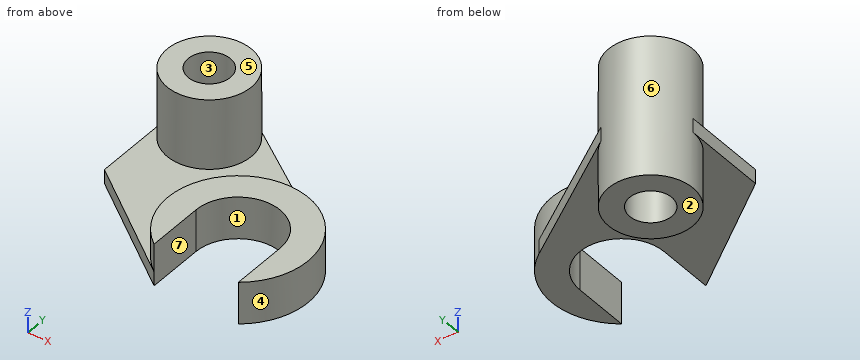
from build123d import *

# Parameters (mm, degrees)
SKETCH1_R                = 30
SKETCH1_R_2              = 15
BOSS_EXTRUDE1_DEPTH      = 50
BOSS_EXTRUDE1_DEPTH_BACK = 50
BOSS_EXTRUDE2_DEPTH      = 20
BOSS_EXTRUDE2_DEPTH_BACK = 10
BOSS_EXTRUDE3_DEPTH      = 10
SKETCH9_R                = 15
CUT_EXTRUDE1_DEPTH       = 51
CUT_EXTRUDE1_DEPTH_BACK  = 51


with BuildPart() as part:
    # Sketch1 → Boss-Extrude1 (new body, two sides)
    with BuildSketch(Plane.XY) as boss_extrude1_sk:
        Circle(SKETCH1_R)
        Circle(SKETCH1_R_2, mode=Mode.SUBTRACT)
    extrude(amount=BOSS_EXTRUDE1_DEPTH)
    extrude(boss_extrude1_sk.sketch, amount=-BOSS_EXTRUDE1_DEPTH_BACK)



with BuildPart() as body_2:
    # Sketch2 → Boss-Extrude2 (new body, two sides)
    with BuildSketch(Plane.XY) as boss_extrude2_sk:
        with BuildLine():
            Line((110, -80), (110, -120))
            ThreePointArc((110, -120), (80, -30), (50, -120))
            Line((50, -120), (50, -80))
            ThreePointArc((50, -80), (80, -50), (110, -80))
        make_face()
    extrude(amount=BOSS_EXTRUDE2_DEPTH)
    extrude(boss_extrude2_sk.sketch, amount=-BOSS_EXTRUDE2_DEPTH_BACK)


with BuildPart() as part_1:
    add(part.part)

    add(body_2.part)  # Boss-Extrude3 merges body 2
    # Sketch3 → Boss-Extrude3 (add)
    with BuildSketch(Plane.XY):
        Polygon((17.129116361, 24.629116361), (108.548527268, -38.951472732), (50, -120), (-30, -60), (-30, 0), align=None)
    extrude(amount=-BOSS_EXTRUDE3_DEPTH)

    # Sketch9 → Cut-Extrude1 (cut, two sides)
    with BuildSketch(Plane.XY) as cut_extrude1_sk:
        Circle(SKETCH9_R)
        with BuildLine():
            Line((50, -80), (50, -120))
            Line((50, -120), (110, -120))
            Line((110, -120), (110, -80))
            ThreePointArc((110, -80), (80, -50), (50, -80))
        make_face()
    extrude(amount=CUT_EXTRUDE1_DEPTH, mode=Mode.SUBTRACT)
    extrude(cut_extrude1_sk.sketch, amount=-CUT_EXTRUDE1_DEPTH_BACK, mode=Mode.SUBTRACT)


solid = part_1.part
Work out the finished part from the listing and answer in its coordinate system (mm). Face numbers are marked on the shaded views. A direction names the side the tool comes from. Give positions to 0.01 mm unless a question says otherwise; leave off trailing zeros. Order: outer loops, then holes, each group sorted by start corner. A loop starts at its lowest first (then second) coordinate and runs counter-clockwise, first axis right, second up. Notation, with made-up numbers: (39.5, 10) - (44.5, 10) arc R20 cw to (44.5, 19) - close; hole circle Ø3 at (88.25, 68). An arc over 180 degrees is marked (long way). Answer as CSV lines item,"result". Start each with the question number.
Q1. Given pin 1 Ø8 at (x, y) = (66.5, -32.5) entering from +Z; pin 2 Ø1.5 at (x, y) = (67, -10) entering from +Z; pin 3 Ø4 at (x, y) = (52, -37) entering from -Z, each flat-ended and moving along its own axis, determine where each tip first touches the part or whether it passes through.
Q2. The part is cut by section D-D (z = 28). Write down the section's boundary in (x, y), then the cut area to 3 significant figures.
Q3. The mould has two halves that part along X. Classify the marked faces 1, 2 and 3: +X half, -X half, draft (parallel to the pull), parting line (faces both ways), or undercut.
Q4. For the marked faces 4, 5, 6 and 7, determine the directions among +Z, -Z, +X, -X, +Y, -Y from which every point of the face is accessible in a straight line to the end or side of a thin tool.
Q5. The part is cut by section B-B (z = 2.5). Write down the section's boundary in (x, y).
Q6. Find the intervals of material crossed by L1, parallel to X at y = 1, z = -19.5; L2, parallel to Y at x = 0, z = 10; L3, parallel to Z at x = 56, y = -16, in increasing order. Write a range as [from, to].
Q7. The part is cut by section A-A (x = 0). Write down the section's boundary in (y, z), then the cut area to 4 significant figures.
Q8. The part is cut by section C-C (y = 6). Write down the section's boundary in (x, z) (3 decimals), then the cut area to 3 significant figures.
Check result:
1,pin 1,"stops at z = 20"
1,pin 2,"stops at z = 0"
1,pin 3,"stops at z = -10"
2,outline,"circle Ø60 at (0, 0); hole circle Ø30 at (0, 0)"
2,area,"2,120 mm²"
3,face 1,"undercut"
3,face 2,"draft"
3,face 3,"undercut"
4,face 4,"+Z"
4,face 5,"+Z, +X, -X, +Y, -Y"
4,face 6,"none"
4,face 7,"+Z, -Z, -Y"
5,outline,"circle Ø60 at (0, 0); (50, -120) - (50, -80) arc R30 cw to (110, -80) - (110, -120) arc R50 ccw (long way) to start; hole circle Ø30 at (0, 0)"
6,L1,"x = [-29.98, -14.97], [14.97, 29.98]"
6,L2,"y = [-30, -15], [15, 30]"
6,L3,"z = [-10, 0]"
7,outline,"(-82.5, -10) - (-30, -10) - (-30, -50) - (-15, -50) - (-15, 50) - (-30, 50) - (-30, 0) - (-82.5, 0) - close; (15, -50) - (30, -50) - (30, 50) - (15, 50) - close"
7,area,"3,525 mm²"
8,outline,"(-29.394, -50) - (-13.748, -50) - (-13.748, 50) - (-29.394, 50) - close; (13.748, -50) - (29.394, -50) - (29.394, -10) - (43.915, -10) - (43.915, 0) - (29.394, 0) - (29.394, 50) - (13.748, 50) - close"
8,area,"3,270 mm²"
